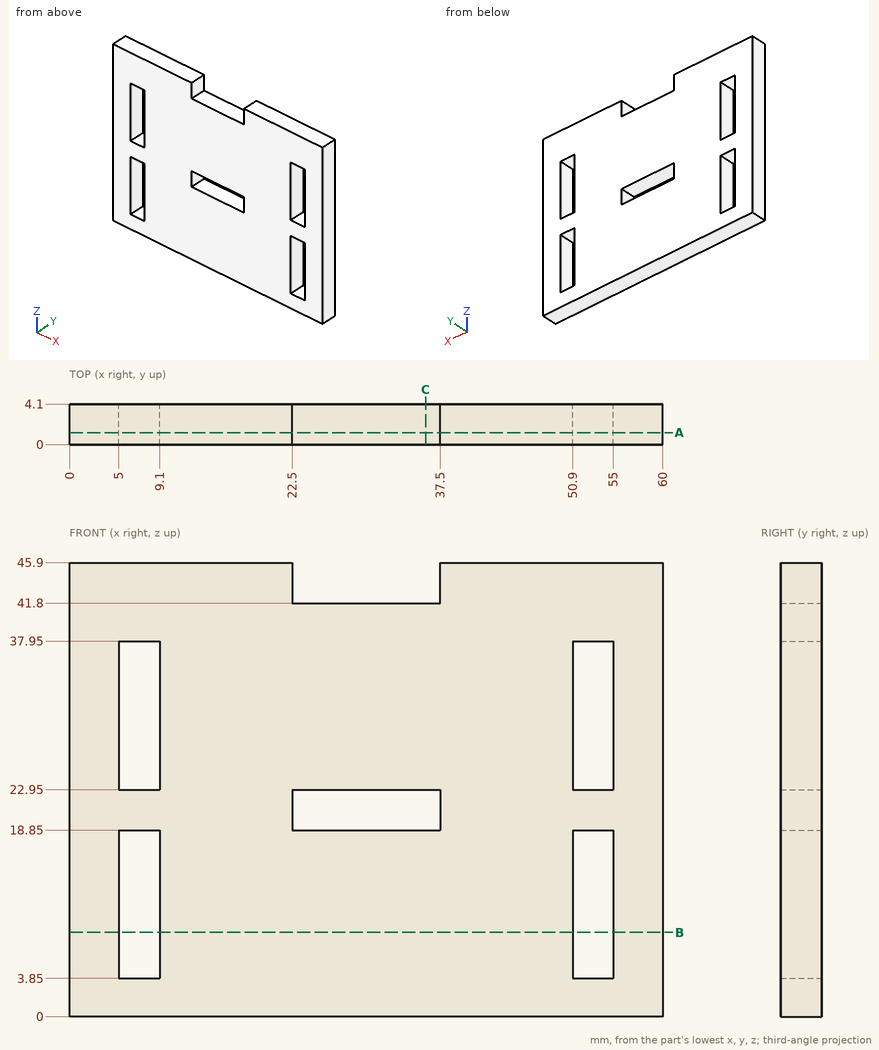
Verification items for this drawing (mm, ordinates from the low corner). Round coordinates to 2 decimals unless told otherwise and drop trailing zeros. Order: outer loops, then holes, each group sorted by start corner. A loop starts at its lowest first (then second) coordinate and runs counter-clockwise, first axis right, second up. Notation, with made-up numbers: (-2, 52.5) -> (50, 52.5) arc R24 ccw to (50, 67.5) -> close; hole circle Ø5 at (-13.5, 73.25). An arc over 180 degrees is marked (long way). Use one line per item in the form item = value.
1. Cross-section at C-C, the plane x = 36. Enter the section's corners in (y, z), plus the area to 3 significant figures.
Working result:
outline = (0, 0) -> (4.1, 0) -> (4.1, 18.85) -> (0, 18.85) -> close; (0, 22.95) -> (4.1, 22.95) -> (4.1, 41.8) -> (0, 41.8) -> close
area = 155 mm^2
2. Go/stop test with flat-tipped pins: pin 1 (5 mm diameter, centred on x = 28, z = 31.5, fed in from -Y); pin 2 (2 mm diameter, centred on x = 33.5, y = 2.5, fed in from +Z). Record where each tip stops, or that it passes through.
Working result:
pin_1 = 0
pin_2 = 41.8
3. Cross-section at B-B, the plane z = 8.5. Enter the section's corners in (x, y), plus the area to 3 significant figures.
Working result:
outline = (0, 0) -> (5, 0) -> (5, 4.1) -> (0, 4.1) -> close; (9.1, 0) -> (50.9, 0) -> (50.9, 4.1) -> (9.1, 4.1) -> close; (55, 0) -> (60, 0) -> (60, 4.1) -> (55, 4.1) -> close
area = 212 mm^2
4. Scan lines: line 1 along X through (y, z) = (3, 35.5); line 2 along X through (y, z) = (1, 21); line 3 along Z through (x, y) = (37, 3.9). Record each from-to range of solid material in increasing order. Write a range as from..to.
Working result:
line_1 = 0..5, 9.1..50.9, 55..60
line_2 = 0..22.5, 37.5..60
line_3 = 0..18.85, 22.95..41.8
5. Cross-section at A-A, the plane y = 1.2. Enter the section's corners in (x, z), plus the area to 4 significant figures.
Working result:
outline = (0, 0) -> (60, 0) -> (60, 45.9) -> (37.5, 45.9) -> (37.5, 41.8) -> (22.5, 41.8) -> (22.5, 45.9) -> (0, 45.9) -> close; hole (5, 3.85) -> (9.1, 3.85) -> (9.1, 18.85) -> (5, 18.85) -> close; hole (5, 22.95) -> (9.1, 22.95) -> (9.1, 37.95) -> (5, 37.95) -> close; hole (22.5, 18.85) -> (37.5, 18.85) -> (37.5, 22.95) -> (22.5, 22.95) -> close; hole (50.9, 3.85) -> (55, 3.85) -> (55, 18.85) -> (50.9, 18.85) -> close; hole (50.9, 22.95) -> (55, 22.95) -> (55, 37.95) -> (50.9, 37.95) -> close
area = 2,385 mm^2
